Geometry: see drawing. Coordinates: mm, zero at the bounding-box minimum. Round coordinates to 2 decimals unless told otherwise and drop trailing zeros. Write each loop counter-clockwise with the first axis right and the second up, starting at its lowest first coordinate (ties: lowest second). Pieces come first, ordered by that corner, then holes. Notation, with made-up numbers: M -40,9 L -14,9 A27 cw -14,42 Z; hole C 86.5,68.5 d6. An arc over 180 degrees is marked long. Use a Markdown table: item, result.
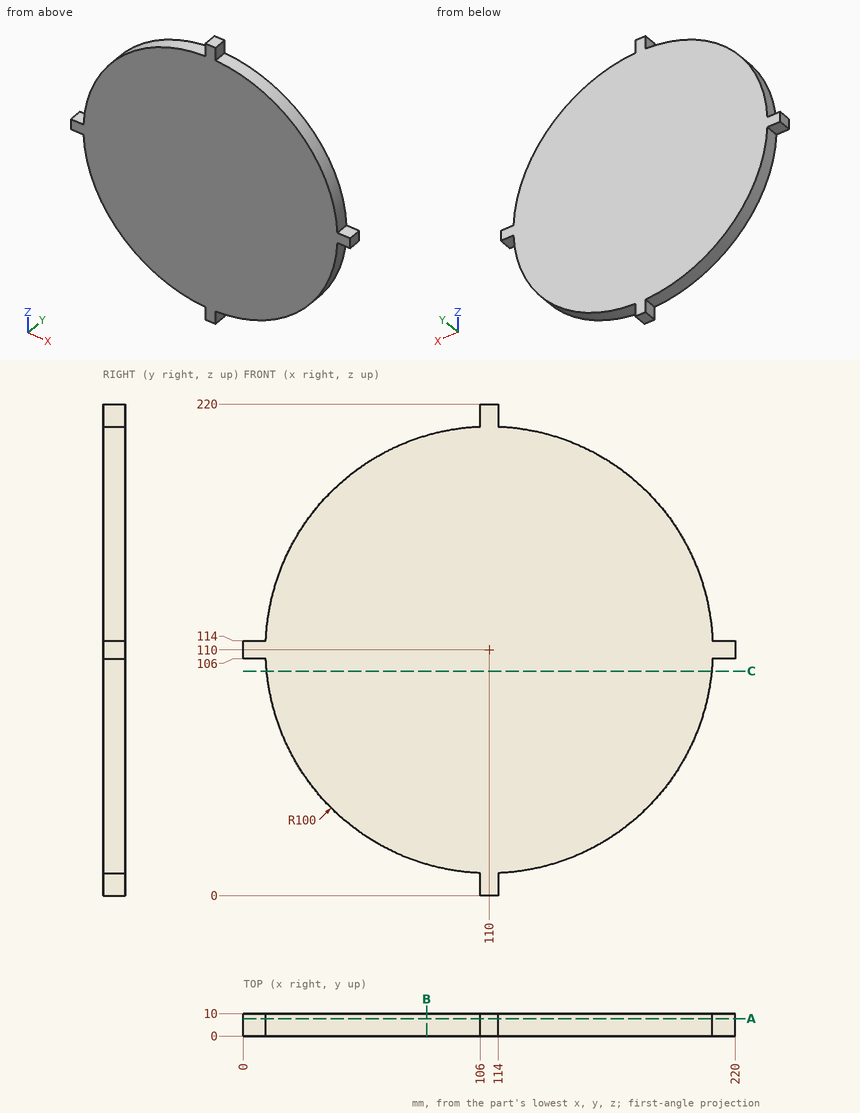
Q1. Section A-A on y = 7.75. Return loops of the section in (x, z).
Results are:
| item | result |
|---|---|
| outline | M 0,106 L 10.08,106 A100 ccw 106,10.08 L 106,0 L 114,0 L 114,10.08 A100 ccw 209.92,106 L 220,106 L 220,114 L 209.92,114 A100 ccw 114,209.92 L 114,220 L 106,220 L 106,209.92 A100 ccw 10.08,114 L 0,114 Z |
Q2. Line query: L1, parallel to X at y = 6.75, z = 146.5; L2, parallel to X at y = 8, z = 70.5; L3, parallel to Z at x = 158, y = 9.5. Output: solid intervals per line, ascending.
Results are:
| item | result |
|---|---|
| L1 | 16.9 to 203.1 |
| L2 | 18.13 to 201.87 |
| L3 | 22.27 to 197.73 |
Q3. Section B-B on x = 82. Return loops of the section in (y, z), plus the area to 3 significant figures.
Results are:
| item | result |
|---|---|
| outline | M 0,14 L 10,14 L 10,206 L 0,206 Z |
| area | 1,920 mm^2 |
Q4. First-contact query: pin 1 Ø1.5 at (x, y) = (61.5, 6.5) entering from -Z; pin 2 Ø3 at (x, y) = (49.5, 5) entering from +Z; pin 3 Ø6 at (x, y) = (72, 6) entering from +Z (3 decimals); pin 4 Ø4 at (x, z) = (29, 46.5) entering from -Y. Flat tips, straight axial feed; report the tip coordinate or a pass-through.
Results are:
| item | result |
|---|---|
| pin 1 | z = 22.14 |
| pin 2 | z = 190.74 |
| pin 3 | z = 203.675 |
| pin 4 | through |
Q5. Section C-C on z = 100.5. Return loops of the section in (x, y), plus the area to 3 significant figures.
Results are:
| item | result |
|---|---|
| outline | M 10.45,0 L 209.55,0 L 209.55,10 L 10.45,10 Z |
| area | 1,990 mm^2 |
